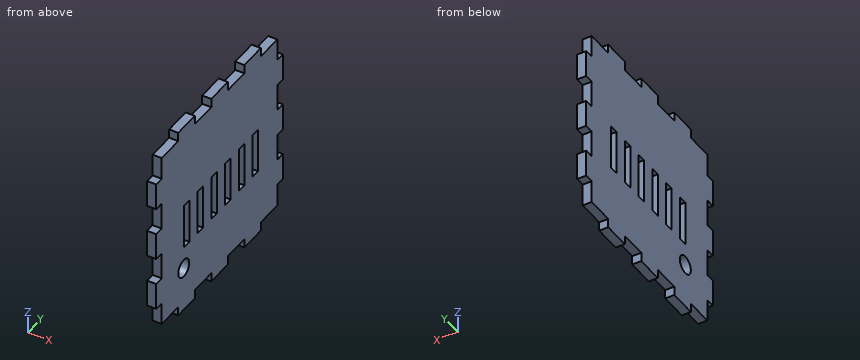
Autodesk Fusion 360 part; units mm, degrees
sketch "スケッチ1" plane through (0, 0, 0) normal (1, 0, 0) x (0, 1, 0)
  line L0 (0, 0) -> (46, 0)
  line L1 (46, 0) -> (46, 44)
  line L2 (46, 44) -> (0, 44)
  line L3 (0, 44) -> (0, 0)
  dimension "d1" = 46
  dimension "d2" = 44
extrude "押し出し1" add sketch "スケッチ1" along normal blind 2
sketch "スケッチ2" plane through (2, 0, 0) normal (1, 0, 0) x (0, 1, 0)
  line L0 (0, 44) -> (0, 0)
  line L1 (0, 0) -> (46, 0)
  line L2 (46, 0) -> (46, 44)
  line L3 (46, 44) -> (0, 44)
  line L4 (0, 0) -> (8, 0)
  line L5 (8, 0) -> (8, 2)
  line L6 (8, 2) -> (0, 2)
  line L7 (0, 2) -> (0, 0)
  line L8 (14, 0) -> (20, 0)
  line L9 (20, 0) -> (20, 2)
  line L10 (20, 2) -> (14, 2)
  line L11 (14, 2) -> (14, 0)
  line L12 (26, 0) -> (32, 0)
  line L13 (32, 0) -> (32, 2)
  line L14 (32, 2) -> (26, 2)
  line L15 (26, 2) -> (26, 0)
  line L16 (46, 0) -> (38, 0)
  line L17 (38, 0) -> (38, 2)
  line L18 (38, 2) -> (46, 2)
  line L19 (46, 2) -> (46, 0)
  line L20 (32, 42) -> (32, 44)
  line L21 (32, 44) -> (26, 44)
  line L22 (20, 42) -> (20, 44)
  line L23 (38, 42) -> (38, 44)
  line L24 (38, 44) -> (46, 44)
  line L25 (46, 44) -> (46, 42)
  line L26 (0, 42) -> (8, 42)
  line L27 (26, 44) -> (26, 42)
  line L28 (8, 42) -> (8, 44)
  line L29 (8, 44) -> (0, 44)
  line L30 (0, 44) -> (0, 42)
  line L31 (20, 44) -> (14, 44)
  line L32 (26, 42) -> (32, 42)
  line L33 (46, 42) -> (38, 42)
  line L34 (14, 42) -> (20, 42)
  line L35 (14, 44) -> (14, 42)
  point P0 (0, 42)
  dimension "d5" = 8
  dimension "d6" = 2
  dimension "d7" = 6
  dimension "d8" = 2
  dimension "d9" = 6
  dimension "d10" = 6
  dimension "d11" = 2
  dimension "d12" = 6
  dimension "d13" = 6
  dimension "d14" = 2
extrude "押し出し2" cut sketch "スケッチ2" against normal blind 2 contours L0 L3 L26 L28 L29 L30 | L0 L1 L4 L5 L6 L7 | L3 L22 L31 L34 L35 | L3 L20 L21 L27 L32 | L1 L8 L9 L10 L11 | L2 L3 L23 L24 L25 L33 | L1 L12 L13 L14 L15 | L1 L2 L16 L17 L18 L19
sketch "スケッチ3" plane through (2, 0, 0) normal (1, 0, 0) x (0, 1, 0)
  line L0 (8, 2) -> (8, 0)
  line L1 (8, 0) -> (14, 0)
  line L2 (14, 0) -> (14, 2)
  line L3 (14, 2) -> (20, 2)
  line L4 (20, 2) -> (20, 0)
  line L5 (20, 0) -> (26, 0)
  line L6 (26, 0) -> (26, 2)
  line L7 (26, 2) -> (32, 2)
  line L8 (32, 2) -> (32, 0)
  line L9 (32, 0) -> (38, 0)
  line L10 (38, 0) -> (38, 2)
  line L11 (38, 2) -> (46, 2)
  line L12 (46, 2) -> (46, 42)
  line L13 (46, 42) -> (38, 42)
  line L14 (38, 42) -> (38, 44)
  line L15 (38, 44) -> (32, 44)
  line L16 (32, 44) -> (32, 42)
  line L17 (32, 42) -> (26, 42)
  line L18 (26, 42) -> (26, 44)
  line L19 (26, 44) -> (20, 44)
  line L20 (20, 44) -> (20, 42)
  line L21 (20, 42) -> (14, 42)
  line L22 (14, 42) -> (14, 44)
  line L23 (14, 44) -> (8, 44)
  line L24 (8, 44) -> (8, 42)
  line L25 (8, 42) -> (0, 42)
  line L26 (0, 42) -> (0, 2)
  line L27 (0, 2) -> (8, 2)
  line L28 (0, 44) -> (2, 44)
  line L29 (2, 44) -> (2, 37)
  line L30 (2, 37) -> (0, 37)
  line L31 (0, 37) -> (0, 44)
  line L32 (2, 31) -> (0, 31)
  line L33 (0, 31) -> (0, 25)
  line L34 (0, 25) -> (2, 25)
  line L35 (2, 25) -> (2, 31)
  line L36 (2, 19) -> (0, 19)
  line L37 (0, 19) -> (0, 13)
  line L38 (0, 13) -> (2, 13)
  line L39 (2, 13) -> (2, 19)
  line L40 (2, 7) -> (0, 7)
  line L41 (0, 7) -> (0, 0)
  line L42 (0, 0) -> (2, 0)
  line L43 (2, 0) -> (2, 7)
  line L44 (46, 31) -> (44, 31)
  line L45 (46, 13) -> (46, 19)
  line L46 (44, 44) -> (46, 44)
  line L47 (44, 0) -> (46, 0)
  line L48 (44, 7) -> (44, 0)
  line L49 (44, 25) -> (46, 25)
  line L50 (46, 37) -> (44, 37)
  line L51 (44, 37) -> (44, 44)
  line L52 (44, 13) -> (46, 13)
  line L53 (44, 31) -> (44, 25)
  line L54 (46, 19) -> (44, 19)
  line L55 (44, 19) -> (44, 13)
  line L56 (46, 25) -> (46, 31)
  line L57 (46, 7) -> (44, 7)
  line L58 (46, 0) -> (46, 7)
  line L59 (46, 44) -> (46, 37)
  point P0 (44, 0)
  dimension "d21" = 2
  dimension "d22" = 7
  dimension "d23" = 2
  dimension "d24" = 6
  dimension "d25" = 6
  dimension "d26" = 6
  dimension "d27" = 6
  dimension "d28" = 2
  dimension "d29" = 6
  dimension "d30" = 7
  dimension "d31" = 2
extrude "押し出し3" cut sketch "スケッチ3" against normal blind 2 contours L27 L41 L42 L43 | L26 L27 L40 L41 L43 | L26 L36 L37 L38 L39 | L26 L32 L33 L34 L35 | L25 L26 L29 L30 L31 | L25 L28 L29 L31 | L11 L12 L48 L57 L58 | L11 L47 L48 L58 | L12 L45 L52 L54 L55 | L12 L44 L49 L53 L56 | L12 L13 L50 L51 L59 | L13 L46 L51 L59
sketch "スケッチ4" plane through (2, 0, 0) normal (1, 0, 0) x (0, 1, 0)
  line L0 (44, 19) -> (46, 19)
  line L1 (46, 19) -> (46, 25)
  line L2 (46, 25) -> (44, 25)
  line L3 (44, 25) -> (44, 31)
  line L4 (44, 31) -> (46, 31)
  line L5 (46, 31) -> (46, 37)
  line L6 (46, 37) -> (44, 37)
  line L7 (44, 37) -> (44, 42)
  line L8 (44, 42) -> (38, 42)
  line L9 (38, 42) -> (38, 44)
  line L10 (38, 44) -> (32, 44)
  line L11 (32, 44) -> (32, 42)
  line L12 (32, 42) -> (26, 42)
  line L13 (26, 42) -> (26, 44)
  line L14 (26, 44) -> (20, 44)
  line L15 (20, 44) -> (20, 42)
  line L16 (20, 42) -> (14, 42)
  line L17 (14, 42) -> (14, 44)
  line L18 (14, 44) -> (8, 44)
  line L19 (8, 44) -> (8, 42)
  line L20 (8, 42) -> (2, 42)
  line L21 (2, 42) -> (2, 37)
  line L22 (2, 37) -> (0, 37)
  line L23 (0, 37) -> (0, 31)
  line L24 (0, 31) -> (2, 31)
  line L25 (2, 31) -> (2, 25)
  line L26 (2, 25) -> (0, 25)
  line L27 (0, 25) -> (0, 19)
  line L28 (0, 19) -> (2, 19)
  line L29 (2, 19) -> (2, 13)
  line L30 (2, 13) -> (0, 13)
  line L31 (0, 13) -> (0, 7)
  line L32 (0, 7) -> (2, 7)
  line L33 (2, 7) -> (2, 2)
  line L34 (2, 2) -> (8, 2)
  line L35 (8, 2) -> (8, 0)
  line L36 (8, 0) -> (14, 0)
  line L37 (14, 0) -> (14, 2)
  line L38 (14, 2) -> (20, 2)
  line L39 (20, 2) -> (20, 0)
  line L40 (20, 0) -> (26, 0)
  line L41 (26, 0) -> (26, 2)
  line L42 (26, 2) -> (32, 2)
  line L43 (32, 2) -> (32, 0)
  line L44 (32, 0) -> (38, 0)
  line L45 (38, 0) -> (38, 2)
  line L46 (38, 2) -> (44, 2)
  line L47 (44, 2) -> (44, 7)
  line L48 (44, 7) -> (46, 7)
  line L49 (46, 7) -> (46, 13)
  line L50 (46, 13) -> (44, 13)
  line L51 (44, 13) -> (44, 19)
  line L52 (10, 15) -> (12, 15)
  line L53 (12, 15) -> (12, 25)
  line L54 (12, 25) -> (10, 25)
  line L55 (10, 25) -> (10, 15)
  line L56 (15, 15) -> (17, 15)
  line L57 (17, 15) -> (17, 25)
  line L58 (17, 25) -> (15, 25)
  line L59 (15, 25) -> (15, 15)
  line L60 (20, 15) -> (22, 15)
  line L61 (22, 15) -> (22, 25)
  line L62 (22, 25) -> (20, 25)
  line L63 (20, 25) -> (20, 15)
  line L64 (25, 15) -> (27, 15)
  line L65 (27, 15) -> (27, 25)
  line L66 (27, 25) -> (25, 25)
  line L67 (25, 25) -> (25, 15)
  line L68 (30, 15) -> (32, 15)
  line L69 (32, 15) -> (32, 25)
  line L70 (32, 25) -> (30, 25)
  line L71 (30, 25) -> (30, 15)
  line L72 (35, 15) -> (37, 15)
  line L73 (37, 15) -> (37, 25)
  line L74 (37, 25) -> (35, 25)
  line L75 (35, 25) -> (35, 15)
extrude "押し出し4" cut sketch "スケッチ4" against normal blind 2 contours L52 L53 L54 L55 | L56 L57 L58 L59 | L60 L61 L62 L63 | L64 L65 L66 L67 | L68 L69 L70 L71 | L72 L73 L74 L75
sketch "スケッチ5" plane through (2, 0, 0) normal (1, 0, 0) x (0, 1, 0)
  line L0 (37, 15) -> (35, 15)
  line L1 (35, 15) -> (35, 25)
  line L2 (35, 25) -> (37, 25)
  line L3 (37, 25) -> (37, 15)
  line L4 (32, 15) -> (30, 15)
  line L5 (30, 15) -> (30, 25)
  line L6 (30, 25) -> (32, 25)
  line L7 (32, 25) -> (32, 15)
  line L8 (17, 15) -> (15, 15)
  line L9 (15, 15) -> (15, 25)
  line L10 (15, 25) -> (17, 25)
  line L11 (17, 25) -> (17, 15)
  line L12 (12, 15) -> (10, 15)
  line L13 (10, 15) -> (10, 25)
  line L14 (10, 25) -> (12, 25)
  line L15 (12, 25) -> (12, 15)
  line L16 (22, 15) -> (20, 15)
  line L17 (20, 15) -> (20, 25)
  line L18 (20, 25) -> (22, 25)
  line L19 (22, 25) -> (22, 15)
  line L20 (27, 15) -> (25, 15)
  line L21 (25, 15) -> (25, 25)
  line L22 (25, 25) -> (27, 25)
  line L23 (27, 25) -> (27, 15)
  line L24 (44, 19) -> (46, 19)
  line L25 (46, 19) -> (46, 25)
  line L26 (46, 25) -> (44, 25)
  line L27 (44, 25) -> (44, 31)
  line L28 (44, 31) -> (46, 31)
  line L29 (46, 31) -> (46, 37)
  line L30 (46, 37) -> (44, 37)
  line L31 (44, 37) -> (44, 42)
  line L32 (44, 42) -> (38, 42)
  line L33 (38, 42) -> (38, 44)
  line L34 (38, 44) -> (32, 44)
  line L35 (32, 44) -> (32, 42)
  line L36 (32, 42) -> (26, 42)
  line L37 (26, 42) -> (26, 44)
  line L38 (26, 44) -> (20, 44)
  line L39 (20, 44) -> (20, 42)
  line L40 (20, 42) -> (14, 42)
  line L41 (14, 42) -> (14, 44)
  line L42 (14, 44) -> (8, 44)
  line L43 (8, 44) -> (8, 42)
  line L44 (8, 42) -> (2, 42)
  line L45 (2, 42) -> (2, 37)
  line L46 (2, 37) -> (0, 37)
  line L47 (0, 37) -> (0, 31)
  line L48 (0, 31) -> (2, 31)
  line L49 (2, 31) -> (2, 25)
  line L50 (2, 25) -> (0, 25)
  line L51 (0, 25) -> (0, 19)
  line L52 (0, 19) -> (2, 19)
  line L53 (2, 19) -> (2, 13)
  line L54 (2, 13) -> (0, 13)
  line L55 (0, 13) -> (0, 7)
  line L56 (0, 7) -> (2, 7)
  line L57 (2, 7) -> (2, 2)
  line L58 (2, 2) -> (8, 2)
  line L59 (8, 2) -> (8, 0)
  line L60 (8, 0) -> (14, 0)
  line L61 (14, 0) -> (14, 2)
  line L62 (14, 2) -> (20, 2)
  line L63 (20, 2) -> (20, 0)
  line L64 (20, 0) -> (26, 0)
  line L65 (26, 0) -> (26, 2)
  line L66 (26, 2) -> (32, 2)
  line L67 (32, 2) -> (32, 0)
  line L68 (32, 0) -> (38, 0)
  line L69 (38, 0) -> (38, 2)
  line L70 (38, 2) -> (44, 2)
  line L71 (44, 2) -> (44, 7)
  line L72 (44, 7) -> (46, 7)
  line L73 (46, 7) -> (46, 13)
  line L74 (46, 13) -> (44, 13)
  line L75 (44, 13) -> (44, 19)
  circle A0 centre (10, 10) radius 2
extrude "押し出し5" cut sketch "スケッチ5" against normal blind 2 contours A0
sketch "スケッチ6" plane through (2, 0, 0) normal (1, 0, 0) x (0, 1, 0)
  circle A0 centre (10, 10) radius 2
  line L0 (37, 15) -> (35, 15)
  line L1 (35, 15) -> (35, 25)
  line L2 (35, 25) -> (37, 25)
  line L3 (37, 25) -> (37, 15)
  line L4 (32, 15) -> (30, 15)
  line L5 (30, 15) -> (30, 25)
  line L6 (30, 25) -> (32, 25)
  line L7 (32, 25) -> (32, 15)
  line L8 (17, 15) -> (15, 15)
  line L9 (15, 15) -> (15, 25)
  line L10 (15, 25) -> (17, 25)
  line L11 (17, 25) -> (17, 15)
  line L12 (12, 15) -> (10, 15)
  line L13 (10, 15) -> (10, 25)
  line L14 (10, 25) -> (12, 25)
  line L15 (12, 25) -> (12, 15)
  line L16 (22, 15) -> (20, 15)
  line L17 (20, 15) -> (20, 25)
  line L18 (20, 25) -> (22, 25)
  line L19 (22, 25) -> (22, 15)
  line L20 (27, 15) -> (25, 15)
  line L21 (25, 15) -> (25, 25)
  line L22 (25, 25) -> (27, 25)
  line L23 (27, 25) -> (27, 15)
  line L24 (44, 19) -> (46, 19)
  line L25 (46, 19) -> (46, 25)
  line L26 (46, 25) -> (44, 25)
  line L27 (44, 25) -> (44, 31)
  line L28 (44, 31) -> (46, 31)
  line L29 (46, 31) -> (46, 37)
  line L30 (46, 37) -> (44, 37)
  line L31 (44, 37) -> (44, 42)
  line L32 (44, 42) -> (38, 42)
  line L33 (38, 42) -> (38, 44)
  line L34 (38, 44) -> (32, 44)
  line L35 (32, 44) -> (32, 42)
  line L36 (32, 42) -> (26, 42)
  line L37 (26, 42) -> (26, 44)
  line L38 (26, 44) -> (20, 44)
  line L39 (20, 44) -> (20, 42)
  line L40 (20, 42) -> (14, 42)
  line L41 (14, 42) -> (14, 44)
  line L42 (14, 44) -> (8, 44)
  line L43 (8, 44) -> (8, 42)
  line L44 (8, 42) -> (2, 42)
  line L45 (2, 42) -> (2, 37)
  line L46 (2, 37) -> (0, 37)
  line L47 (0, 37) -> (0, 31)
  line L48 (0, 31) -> (2, 31)
  line L49 (2, 31) -> (2, 25)
  line L50 (2, 25) -> (0, 25)
  line L51 (0, 25) -> (0, 19)
  line L52 (0, 19) -> (2, 19)
  line L53 (2, 19) -> (2, 13)
  line L54 (2, 13) -> (0, 13)
  line L55 (0, 13) -> (0, 7)
  line L56 (0, 7) -> (2, 7)
  line L57 (2, 7) -> (2, 2)
  line L58 (2, 2) -> (8, 2)
  line L59 (8, 2) -> (8, 0)
  line L60 (8, 0) -> (14, 0)
  line L61 (14, 0) -> (14, 2)
  line L62 (14, 2) -> (20, 2)
  line L63 (20, 2) -> (20, 0)
  line L64 (20, 0) -> (26, 0)
  line L65 (26, 0) -> (26, 2)
  line L66 (26, 2) -> (32, 2)
  line L67 (32, 2) -> (32, 0)
  line L68 (32, 0) -> (38, 0)
  line L69 (38, 0) -> (38, 2)
  line L70 (38, 2) -> (44, 2)
  line L71 (44, 2) -> (44, 7)
  line L72 (44, 7) -> (46, 7)
  line L73 (46, 7) -> (46, 13)
  line L74 (46, 13) -> (44, 13)
  line L75 (44, 13) -> (44, 19)
Check sheet for the modelled part. Datum: model origin and axes. Units: mm. Round coordinates to 2 decimals unless told otherwise and drop trailing zeros. Order: outer loops, then holes, each group sorted by start corner. A loop starts at its lowest first (then second) coordinate and runs counter-clockwise, first axis right, second up. Notation, with made-up numbers: (85, -29.5) - (101, -29.5) arc R21 ccw to (101, -20.5) - close; hole circle Ø7 at (-13, 25.25). An arc over 180 degrees is marked (long way). Answer as CSV lines item,"result". Start each with the question number.
1) Section check A-A (z = 10). Record the cut outline in (x, y).
2) Depth check by flat-ended pin: pin 1 (0.6 mm diameter, centred on x = 1, z = 39.5, fed in from +Y); pin 2 (2 mm diameter, centred on y = 38, z = 16.5, fed in from -X); pin 3 (1 mm diameter, centred on x = 1, y = 42, fed in from +Z); pin 4 (1 mm diameter, centred on x = 1, y = 45, fed in from -Z). Enter the tip coordinate at first touch or a pass-through.
3) Scan lines: probe 1 along Y at (x, z) = (0.6, 42.5); probe 2 along Z at (x, y) = (1.4, 21.5); probe 3 along Y at (x, z) = (0.65, 27.5). Record each from-to range of solid material in increasing order.
4) Section check B-B (x = 0.5). Give the number of separate pieces and of enclosed holes in the cut face, then the cut area to 3 significant figures.
5) Section check C-C (y = 41). Record the cut outline in (x, z).
Determined:
1,outline,"(0, 0) - (2, 0) - (2, 8) - (0, 8) - close; (0, 12) - (2, 12) - (2, 46) - (0, 46) - close"
2,pin 1,"y = 44"
2,pin 2,"x = 0"
2,pin 3,"z = 42"
2,pin 4,"z = 7"
3,probe 1,"8 to 14, 20 to 26, 32 to 38"
3,probe 2,"0 to 15, 25 to 44"
3,probe 3,"2 to 44"
4,separate pieces,"1"
4,enclosed holes,"7"
4,area,"1,690 mm^2"
5,outline,"(0, 2) - (2, 2) - (2, 42) - (0, 42) - close"
